For this review, take the finished solid that the model builds, in its own axes (mm). A direction names the side the tool comes from. Coordinates: 2 decimals unless noted, no trailing zeros. Order: outer loops, then holes, each group sorted by start corner. A loop starts at its lowest first (then second) coordinate and runs counter-clockwise, first axis right, second up. Notation, with made-up numbers: (-26, 22) -> (12, 22) arc R8 cw to (12, 34) -> close; hole circle Ø10 at (86.5, -11.75). An arc over 180 degrees is marked (long way). Answer as a JSON object with one key per item and string values. Group by question number.
1) Add section D-D, the plane z = 96. Write out the cut boundary in (x, y), then the cut area to 3 significant figures.
2) Add section C-C, the plane y = 57.5. Write out the cut boundary in (x, z), then the cut area to 3 significant figures.
3) For pin 1 (2.5 mm diameter, centred on x = 64.5, z = 88, fed in from -Y); pin 2 (1.5 mm diameter, centred on x = 5, y = 67.5, fed in from +Z); pin 3 (1.7 mm diameter, centred on y = 55.5, z = 96.5, fed in from -X); pin 4 (2 mm diameter, centred on x = 39.5, y = 77, fed in from +Z), all flat-tipped, find the tip position at first contact; note any pin that passes through.
4) Wall thickness on L1, parallel to X at y = 67, z = 92; L2, parallel to X at y = 67, z = 100; L3, parallel to Z at x = 34.5, y = 55.5: over which ranges is each line inside the solid? List them lowest first.
5) Machinability: for faces 1 (the flat face through (-5.017, 56, 101)), 2 (the cylindrical face through (-6.64, 71.02, 64.203)), 3 (the flat face through (29, 54.968, 101)), 4 (the flat face through (29, 80, 92.077)), which of the approach directions +Z, -Z, +X, -X, +Y, -Y give a long, thin tool a straight path to every point of the face, cutting with its end or side? Answer none if there is none.
6) Add section B-B, the plane z = 83. Write out the cut boundary in (x, y).
7) Draft analysis for pull direction Y (two halves, no side actions). For faces 5 (the flat face through (58.183, 70, 101)), 6 (the cylindrical face through (-6.64, 69.43, 54.93)), 7 (the flat face through (64, 58.918, 88)), state which applies: +Y half, -Y half, draft (parallel to the pull), parting line (faces both ways), or undercut.
8) Add section A-A, the plane x = 26. Write out the cut boundary in (y, z).
from build123d import *

# Parameters (mm, degrees)
SKETCH_2_R          = 1.6
SKETCH_2_R_2        = 0.5
BOSS_EXTRUDE1_DEPTH = 3.2
SKETCH1_W           = 18.6
SKETCH1_H           = 33
SKETCH1_W_2         = 16
SKETCH1_H_2         = 29.4
BOSS_EXTRUDE2_DEPTH = 67.4
CUT_EXTRUDE1_REACH  = 116.482
SKETCH2_W           = 42.896922538
SKETCH2_H           = 18.367032987
CUT_EXTRUDE2_REACH  = 123.795
SKETCH3_W           = 27
SKETCH3_H           = 17
BOSS_EXTRUDE3_START = 3.2
BOSS_EXTRUDE3_DEPTH = 3.2
SKETCH5_R           = 2
CUT_EXTRUDE3_DEPTH  = 10
SKETCH6_W           = 16
SKETCH6_H           = 29.4
BOSS_EXTRUDE4_DEPTH = 4.2
SKETCH7_W           = 16
SKETCH7_H           = 29.4
BOSS_EXTRUDE5_DEPTH = 4.2
CUT_EXTRUDE5_DEPTH  = 30


with BuildPart() as part:
    # 스케치2 → Boss-Extrude1 (new body)
    with BuildSketch(Plane(origin=(62.38287134, 0, 0), x_dir=(0, 0, -1), z_dir=(1, 0, 0))):
        with BuildLine():
            Line((-65.677419436, 80.41810471), (-110.677419436, 80.41810471))
            Line((-110.677419436, 80.41810471), (-110.677419436, 58.91810471))
            Line((-110.677419436, 58.91810471), (-65.677419436, 58.91810471))
            ThreePointArc((-65.677419436, 58.91810471), (-54.927419436, 69.66810471), (-65.677419436, 80.41810471))
        make_face()
        with Locations((-66.314714345, 62.596764299)):
            Circle(SKETCH_2_R, mode=Mode.SUBTRACT)
        with Locations((-61.803243354, 76.447725619)):
            Circle(SKETCH_2_R_2, mode=Mode.SUBTRACT)
        with Locations((-68.277005701, 77.03116462)):
            Circle(SKETCH_2_R_2, mode=Mode.SUBTRACT)
        with Locations((-72.457040346, 73.542280792)):
            Circle(SKETCH_2_R_2, mode=Mode.SUBTRACT)
        with Locations((-72.748759847, 70.305399618)):
            Circle(SKETCH_2_R_2, mode=Mode.SUBTRACT)
        with Locations((-73.040479347, 67.068518444)):
            Circle(SKETCH_2_R_2, mode=Mode.SUBTRACT)
        with Locations((-69.551595519, 62.8884838)):
            Circle(SKETCH_2_R_2, mode=Mode.SUBTRACT)
        with Locations((-63.077833171, 62.305044799)):
            Circle(SKETCH_2_R_2, mode=Mode.SUBTRACT)
        with Locations((-58.897798526, 65.793928627)):
            Circle(SKETCH_2_R_2, mode=Mode.SUBTRACT)
        with Locations((-58.606079026, 69.030809801)):
            Circle(SKETCH_2_R_2, mode=Mode.SUBTRACT)
        with Locations((-58.314359525, 72.267690975)):
            Circle(SKETCH_2_R_2, mode=Mode.SUBTRACT)
        with Locations((-65.040124528, 76.73944512)):
            Circle(SKETCH_2_R, mode=Mode.SUBTRACT)
    extrude(amount=BOSS_EXTRUDE1_DEPTH)

    # Sketch1 → Boss-Extrude2 (add)
    with BuildSketch(Plane.ZY.offset(-62.38287134)):
        with Locations((101.377419436, 69.66810471)):
            Rectangle(SKETCH1_W, SKETCH1_H)
        with Locations((101.077419436, 69.66810471)):
            Rectangle(SKETCH1_W_2, SKETCH1_H_2, mode=Mode.SUBTRACT)
    extrude(amount=BOSS_EXTRUDE2_DEPTH)

    # Sketch2 → Cut-Extrude1 (cut, up to next)
    with BuildSketch(Plane(origin=(0, 0, 92.077419436), x_dir=(-1, 0, 0), z_dir=(0, 0, -1)), mode=Mode.PRIVATE) as cut_extrude1_sk1:
        with Locations((-28.68287134, 69.668104709)):
            Rectangle(SKETCH2_W, SKETCH2_H)
    cut_extrude1_tool1 = extrude(cut_extrude1_sk1.sketch, amount=-CUT_EXTRUDE1_REACH, mode=Mode.PRIVATE) & part.part
    add(cut_extrude1_tool1.solids().sort_by_distance((28.682871, 69.668105, 92.077419))[0], mode=Mode.SUBTRACT)

    # Sketch3 → Cut-Extrude2 (cut, up to next)
    with BuildSketch(Plane.XY.offset(110.677419436), mode=Mode.PRIVATE) as cut_extrude2_sk1:
        with Locations((28.68287134, 69.66810471)):
            Rectangle(SKETCH3_W, SKETCH3_H)
    cut_extrude2_tool1 = extrude(cut_extrude2_sk1.sketch, amount=-CUT_EXTRUDE2_REACH, mode=Mode.PRIVATE) & part.part
    add(cut_extrude2_tool1.solids().sort_by_distance((28.682871, 69.668105, 110.677419))[0], mode=Mode.SUBTRACT)

    # Sketch4 → Boss-Extrude3 (add)
    with BuildSketch(Plane.ZY.offset(5.01712866).offset(BOSS_EXTRUDE3_START)):
        with BuildLine():
            Line((65.677419436, 80.41810471), (110.677419436, 80.41810471))
            Line((110.677419436, 80.41810471), (110.677419436, 58.91810471))
            Line((110.677419436, 58.91810471), (65.677419436, 58.91810471))
            ThreePointArc((65.677419436, 58.91810471), (54.927419436, 69.66810471), (65.677419436, 80.41810471))
        make_face()
    extrude(amount=-BOSS_EXTRUDE3_DEPTH)

    # Sketch5 → Cut-Extrude3 (cut)
    with BuildSketch(Plane.ZY.offset(8.21712866)):
        with Locations((65.677419436, 69.66810471)):
            Circle(SKETCH5_R)
    extrude(amount=-CUT_EXTRUDE3_DEPTH, mode=Mode.SUBTRACT)

    # Sketch6 → Boss-Extrude4 (add)
    with BuildSketch(Plane(origin=(62.38287134, 0, 0), x_dir=(0, 0, -1), z_dir=(1, 0, 0))):
        with Locations((-101.077419436, 69.66810471)):
            Rectangle(SKETCH6_W, SKETCH6_H)
    extrude(amount=-BOSS_EXTRUDE4_DEPTH)

    # Sketch7 → Boss-Extrude5 (add)
    with BuildSketch(Plane.ZY.offset(5.01712866)):
        with Locations((101.077419436, 69.66810471)):
            Rectangle(SKETCH7_W, SKETCH7_H)
    extrude(amount=-BOSS_EXTRUDE5_DEPTH)

    # Sketch10 → Cut-Extrude5 (cut)
    with BuildSketch(Plane(origin=(0, 86.16810471, 0), x_dir=(1, 0, 0), z_dir=(0, 1, 0))):
        Polygon((-1.81712866, -110.677419436), (59.18287134, -110.677419436), (59.18287134, -109.677419436), (59.88287134, -109.677419436), (59.88287134, -109.077419436), (-2.51712866, -109.077419436), (-2.51712866, -109.677419436), (-1.81712866, -109.677419436), align=None)
    extrude(amount=-CUT_EXTRUDE5_DEPTH, mode=Mode.SUBTRACT)


solid = part.part
Output values:
{
 "1": {"outline": "(-8.22, 58.92) -> (-5.02, 58.92) -> (-5.02, 53.17) -> (62.38, 53.17) -> (62.38, 58.92) -> (65.58, 58.92) -> (65.58, 80.42) -> (62.38, 80.42) -> (62.38, 86.17) -> (-5.02, 86.17) -> (-5.02, 80.42) -> (-8.22, 80.42) -> close; hole (-0.82, 54.97) -> (58.18, 54.97) -> (58.18, 84.37) -> (-0.82, 84.37) -> close", "area": "627 mm²"},
 "2": {"outline": "(-5.02, 92.08) -> (62.38, 92.08) -> (62.38, 110.68) -> (59.18, 110.68) -> (59.18, 109.68) -> (59.88, 109.68) -> (59.88, 109.08) -> (58.18, 109.08) -> (58.18, 93.08) -> (-0.82, 93.08) -> (-0.82, 109.08) -> (-2.52, 109.08) -> (-2.52, 109.68) -> (-1.82, 109.68) -> (-1.82, 110.68) -> (-5.02, 110.68) -> close", "area": "211 mm²"},
 "3": {"pin 1": "stops at y = 58.92", "pin 2": "stops at z = 93.08", "pin 3": "stops at x = -5.02", "pin 4": "passes through"},
 "4": {"L1": "x = -8.22 to -5.02, 62.38 to 65.58", "L2": "x = -8.22 to -0.82, 58.18 to 65.58", "L3": "z = 92.08 to 93.08, 109.08 to 110.68"},
 "5": {"face 1": "+Z, -Z, -X, -Y", "face 2": "-X", "face 3": "none", "face 4": "-Z, +Y, -Y"},
 "6": {"outline": "(-8.22, 58.92) -> (-5.02, 58.92) -> (-5.02, 80.42) -> (-8.22, 80.42) -> close; (62.38, 58.92) -> (65.58, 58.92) -> (65.58, 80.42) -> (62.38, 80.42) -> close"},
 "7": {"face 5": "undercut", "face 6": "parting line", "face 7": "-Y half"},
 "8": {"outline": "(53.17, 92.08) -> (60.48, 92.08) -> (60.48, 93.08) -> (54.97, 93.08) -> (54.97, 109.08) -> (56.17, 109.08) -> (56.17, 110.68) -> (53.17, 110.68) -> close; (78.85, 92.08) -> (86.17, 92.08) -> (86.17, 109.08) -> (84.37, 109.08) -> (84.37, 93.08) -> (78.85, 93.08) -> close"}
}
